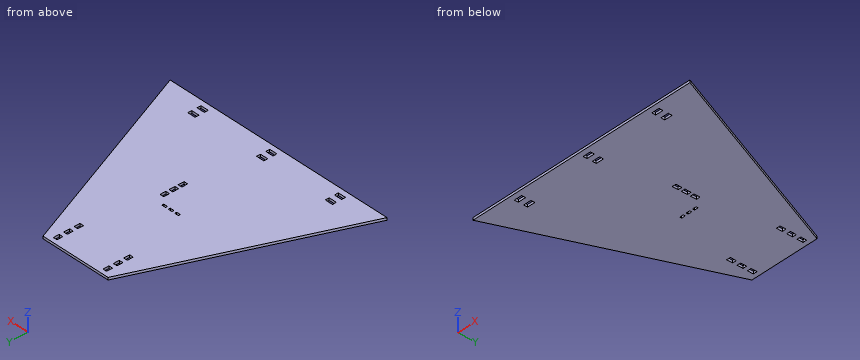
```python
from build123d import *

# Parameters (mm, degrees)
SKETCH1_W           = 20
SKETCH1_H           = 10
SKETCH1_W_2         = 10
SKETCH1_H_2         = 5
SKETCH1_H_3         = 15
BOSS_EXTRUDE1_DEPTH = 6


with BuildPart() as part:
    # Sketch1 → Boss-Extrude1 (new body)
    with BuildSketch(Plane.XY):
        Polygon((296.475, 0), (0, 0), (210.025, 514.3036198), (390.025, 514.3036198), (600.05, 0), (300.025, 0), align=None)
        with Locations((110, 18.333333333)):
            Rectangle(SKETCH1_W, SKETCH1_H, mode=Mode.SUBTRACT)
        with Locations((110, 41.666666667)):
            Rectangle(SKETCH1_W, SKETCH1_H, mode=Mode.SUBTRACT)
        with Locations((490.05, 41.666666667)):
            Rectangle(SKETCH1_W, SKETCH1_H, mode=Mode.SUBTRACT)
        with Locations((490.05, 18.333333333)):
            Rectangle(SKETCH1_W, SKETCH1_H, mode=Mode.SUBTRACT)
        with Locations((308.575, 280.6998099)):
            Rectangle(SKETCH1_W_2, SKETCH1_H_2, mode=Mode.SUBTRACT)
        with Locations((290.825, 280.6998099)):
            Rectangle(SKETCH1_W_2, SKETCH1_H_2, mode=Mode.SUBTRACT)
        with Locations((273.075, 280.6998099)):
            Rectangle(SKETCH1_W_2, SKETCH1_H_2, mode=Mode.SUBTRACT)
        with Locations((368.725, 495.5536198)):
            Rectangle(SKETCH1_W_2, SKETCH1_H_3, mode=Mode.SUBTRACT)
        with Locations((368.725, 469.3036198)):
            Rectangle(SKETCH1_W_2, SKETCH1_H_3, mode=Mode.SUBTRACT)
        with Locations((336.325, 255.0068099)):
            Rectangle(SKETCH1_W_2, SKETCH1_H_3, mode=Mode.SUBTRACT)
        with Locations((336.325, 232.0068099)):
            Rectangle(SKETCH1_W_2, SKETCH1_H_3, mode=Mode.SUBTRACT)
        with Locations((336.325, 209.0068099)):
            Rectangle(SKETCH1_W_2, SKETCH1_H_3, mode=Mode.SUBTRACT)
        with Locations((368.725, 443.0536198)):
            Rectangle(SKETCH1_W_2, SKETCH1_H_3, mode=Mode.SUBTRACT)
        with Locations((231.325, 443.0536198)):
            Rectangle(SKETCH1_W_2, SKETCH1_H_3, mode=Mode.SUBTRACT)
        with Locations((231.325, 469.3036198)):
            Rectangle(SKETCH1_W_2, SKETCH1_H_3, mode=Mode.SUBTRACT)
        with Locations((231.325, 495.5536198)):
            Rectangle(SKETCH1_W_2, SKETCH1_H_3, mode=Mode.SUBTRACT)
        with Locations((300.025, 41.666666667)):
            Rectangle(SKETCH1_W, SKETCH1_H, mode=Mode.SUBTRACT)
        with Locations((300.025, 18.333333333)):
            Rectangle(SKETCH1_W, SKETCH1_H, mode=Mode.SUBTRACT)
    extrude(amount=BOSS_EXTRUDE1_DEPTH)


solid = part.part
```
Can you work these out from the model? Positions are in its coordinate system, mm. Coordinates: 2 decimals unless noted, no trailing zeros. Write each loop counter-clockwise with the first axis right and the second up, starting at its lowest first coordinate (ties: lowest second). Pieces come first, ordered by that corner, then holes. Notation, with made-up numbers: M 60.5,0 L 97.5,0 A16 cw 97.5,27 Z; hole C -37,-23 d6. An arc over 180 degrees is marked long. Write item = value, one per line. Start each with the question number.
Q1. If we section it at A-A, the plane y = 209.5: Write out the boundary of the cut face in (x, z) (3 decimals), then the cut area to 3 significant figures.
Q2. If we section it at B-B, the plane z = 3.15: State how many separate pieces and enclosed holes the cut face has, then the cut area to 3 significant figures.
Q3. If we section it at C-C, the plane x = 537.5: Write out the boundary of the cut face in (y, z).
Q4. If I drill on L1, parallel to Y at x = 364, z = 3.4; L2, parallel to Y at x = 271.5, z = 3.2; L3, parallel to X at y = 475, z = 1.4 (3 decimals), over which ranges is the centre line in solid material (lowest first)? Write a range as [from, to].
Q5. If we section it at D-D, the plane x = 139: Write out the boundary of the cut face in (y, z).
Q6. I'm going to push flat-ended pins straight in: pin 1 (3 mm diameter, centred on y = 472.5, z = 3.5, fed in from +X); pin 2 (1.8 mm diameter, centred on x = 112, z = 4.5, fed in from +Y); pin 3 (3 mm diameter, centred on y = 255.5, z = 2, fed in from -X). Where does each tip first touch, or does it pass through?
Check sheet entries:
q1.outline = M 85.553,0 L 331.325,0 L 331.325,6 L 85.553,6 Z; M 341.325,0 L 514.497,0 L 514.497,6 L 341.325,6 Z
q1.area = 2,510 mm²
q2.separate_pieces = 1
q2.enclosed_holes = 18
q2.area = 198,000 mm²
q3.outline = M 0,0 L 153.17,0 L 153.17,6 L 0,6 Z
q4.L1 = [0, 435.55], [450.55, 461.8], [476.8, 488.05], [503.05, 514.3]
q4.L2 = [0, 278.2], [283.2, 514.3]
q4.L3 = [193.975, 226.325], [236.325, 363.725], [373.725, 406.075]
q5.outline = M 0,0 L 340.38,0 L 340.38,6 L 0,6 Z
q6.pin_1 = 407.71
q6.pin_2 = 276.47
q6.pin_3 = 103.73
